Could you check a few things on this model? Use its own coordinates, in mm. Face numbers are marked on the shaded views. A direction names the side the tool comes from. Give positions to 0.01 mm unless a question says otherwise; leave off trailing zeros. Write each loop counter-clockwise with the first axis right and the second up, starting at its lowest first coordinate (ties: lowest second). Pieces come first, ordered by that corner, then holes. Notation, with made-up numbers: (65.5, -39) -> (119.5, -39) arc R20 cw to (119.5, -13) -> close; hole circle Ø6 at (59.25, 26.25). An arc over 180 degrees is marked (long way). One line per question, with ' | ' between items.
from build123d import *

# Parameters (mm, degrees)
F1_DEPTH = 12.7
F2_W     = 25.4
F2_H     = 76.2
F3_DEPTH = 12.7
F4_W     = 50.8
F4_H     = 76.2
F5_DEPTH = 12.7
F7_DEPTH = 12.7


with BuildPart() as f1:
    # F0 (on Top) → F1 (new body)
    with BuildSketch(Plane.XY):
        Polygon((-42.839443, 47.784637), (-68.239443, 47.784637), (-68.239443, -28.415363), (-42.839443, -28.415363), (7.960557, -28.415363), (58.760557, -28.415363), (58.760557, 47.784637), (7.960557, 47.784637), align=None)
    extrude(amount=F1_DEPTH)

    # F2 (on face) → F3 (join)
    with BuildSketch(Plane.XY.offset(12.7)):
        with Locations((-55.539443, 9.684637)):
            Rectangle(F2_W, F2_H)
    extrude(amount=F3_DEPTH)

    # F4 (on face) → F5 (join)
    with BuildSketch(Plane.XY.offset(12.7)):
        with Locations((33.360557, 9.684637)):
            Rectangle(F4_W, F4_H)
    extrude(amount=F5_DEPTH)

    # F6 (on face) → F7 (join)
    with BuildSketch(Plane(origin=(0, 0, 0), x_dir=(1, 0, 0), z_dir=(0, 0, -1))):
        with BuildLine():
            Line((27.010557, 17.746579), (-4.739443, 17.746579))
            Line((-4.739443, 17.746579), (-36.489443, 17.746579))
            Line((-36.489443, 17.746579), (-36.489443, 0))
            Line((-36.489443, 0), (-36.489443, -6.262278))
            ThreePointArc((-36.489443, -6.262278), (-26.403608, -28.083061), (-4.739443, -38.501054))
            ThreePointArc((-4.739443, -38.501054), (16.924722, -28.083061), (27.010557, -6.262278))
            Line((27.010557, -6.262278), (27.010557, 0))
            Line((27.010557, 0), (27.010557, 17.746579))
        make_face()
    extrude(amount=F7_DEPTH)


solid = f1.part
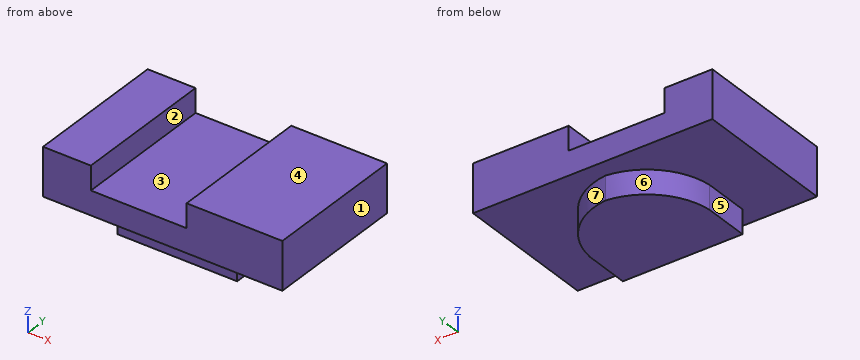
Q1. Imagine slicing it at B-B on y = -5. Please give me the cut outline in (x, z).
Answer below:
outline: (-68.24, 0) -> (-36.49, 0) -> (-36.49, -12.7) -> (27.01, -12.7) -> (27.01, 0) -> (58.76, 0) -> (58.76, 25.4) -> (7.96, 25.4) -> (7.96, 12.7) -> (-42.84, 12.7) -> (-42.84, 25.4) -> (-68.24, 25.4) -> close
Q2. Imagine slicing it at A-A on z = 22. Please give me the cut outline in (x, y).
Answer below:
outline: (-68.24, -28.42) -> (-42.84, -28.42) -> (-42.84, 47.78) -> (-68.24, 47.78) -> close; (7.96, -28.42) -> (58.76, -28.42) -> (58.76, 47.78) -> (7.96, 47.78) -> close
Q3. On a 3-axis mill with a long thin cutter (end or side, diameter ignored), from which of +Z, -Z, +X, -X, +Y, -Y can I reach the whole of each face in a straight line? I mean the marked faces 5, 6 and 7. Say none if no direction works.
Answer below:
face 5: -Z, -X, +Y, -Y | face 6: -Z, -X, +Y | face 7: -Z, +X, +Y
Q4. If we mould it in two halves opening along X, with no side actions, what happens to the marked faces 1, 2, 3 and 4? For each: +X half, -X half, draft (parallel to the pull), parting line (faces both ways), or undercut.
Answer below:
face 1: +X half | face 2: undercut | face 3: undercut | face 4: draft
Q5. Imagine slicing it at D-D on x = 20. Please give me the cut outline in (y, z).
Answer below:
outline: (-28.42, 0) -> (-17.75, 0) -> (-17.75, -12.7) -> (24.52, -12.7) -> (24.52, 0) -> (47.78, 0) -> (47.78, 25.4) -> (-28.42, 25.4) -> close
Q6. If I drill on line 1 along X through (y, z) = (5, 20); line 2 along Z through (x, y) = (-1, -2); line 3 along Z through (x, y) = (-6, -20.5), over which ranges is the centre line in solid material (lowest first)?
Answer below:
line 1: x = -68.24 to -42.84, 7.96 to 58.76 | line 2: z = -12.7 to 12.7 | line 3: z = 0 to 12.7
Q7. Will these pins go through, and if not, where does the flat tip stop? pin 1 (4 mm diameter, centred on x = -12, z = -8.5, fed in from -Y); pin 2 (10 mm diameter, centred on y = -7.5, z = -6, fed in from +X); pin 3 (8 mm diameter, centred on y = 14, z = -7, fed in from +X).
Answer below:
pin 1: stops at y = -17.75 | pin 2: stops at x = 27.01 | pin 3: stops at x = 26.48
Q8. Imagine slicing it at C-C on z = -8. Please give me the cut outline in (x, y).
Answer below:
outline: (-36.49, -17.75) -> (27.01, -17.75) -> (27.01, 6.26) arc R35.56 ccw to (-4.74, 38.5) arc R35.56 ccw to (-36.49, 6.26) -> close
